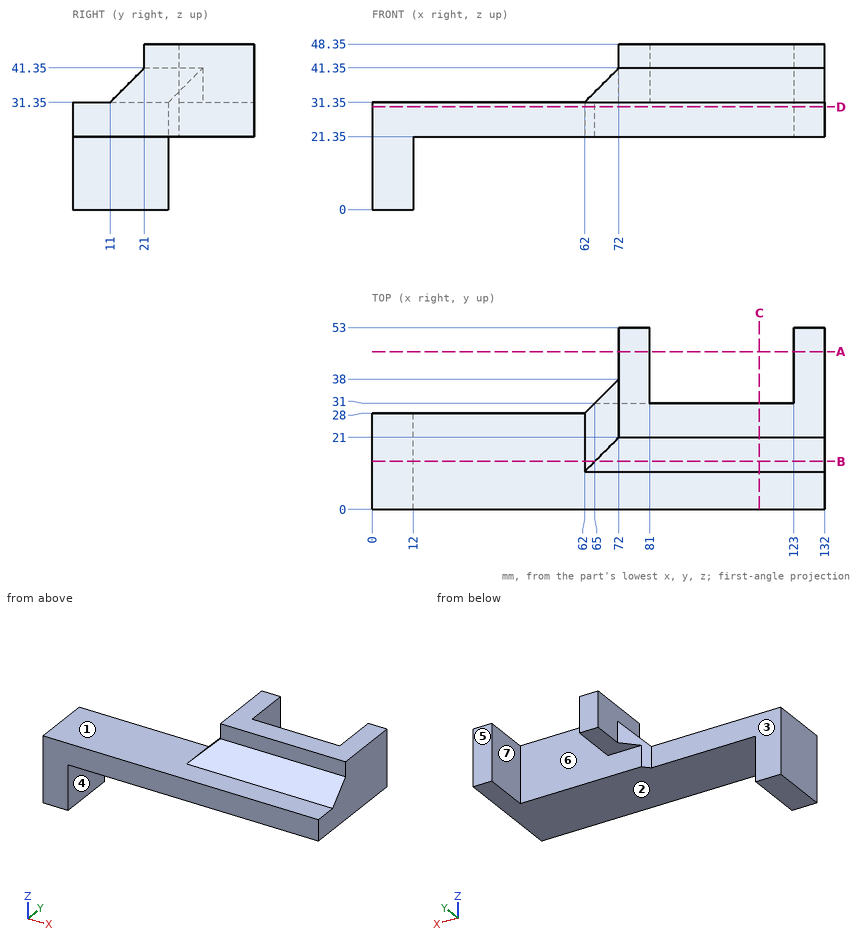
Design review of the part shown in the three views and the two pictorial views. Dimensions are in mm from the part's minimum x, y and z. A direction names the side the tool comes from. Round coordinates to 2 decimals unless told otherwise and drop trailing zeros. Loops run counter-clockwise (first coordinate to the right, second up) from the corner with the lowest first, then second, coordinate; pieces in that order, holes last.
1) Consider section B-B on y = 14. State the section outline as (x, z) points, then the cut area to 3 significant figures.
Values follow:
outline: (0, 0) - (12, 0) - (12, 21.35) - (132, 21.35) - (132, 34.35) - (65, 34.35) - (62, 31.35) - (0, 31.35) - close
area: 1,780 mm2
2) Wall thickness on line 1 along Z through (x, y) = (32, 27.5); line 2 along Z through (x, y) = (9, 6.5); line 3 along X through (y, z) = (23, 43): over which ranges is each line inside the solid? List them lowest first.
Values follow:
line 1: z = 21.35 to 31.35
line 2: z = 0 to 31.35
line 3: x = 72 to 132
3) Consider section C-C on x = 113. State the section outline as (y, z) points.
Values follow:
outline: (0, 21.35) - (31, 21.35) - (31, 48.35) - (21, 48.35) - (21, 41.35) - (11, 31.35) - (0, 31.35) - close
4) Clearance check with flat-ended pins moving along their axes: P1, Ø8.5, axis at x = 88.5, y = 10, coming from the +Z side; P2, Ø7.5, axis at x = 98.5, z = 45.5, coming from the -Y side; P3, Ø13, axis at x = 73, y = 42, coming from the -Z side; P4, Ø2, axis at y = 14, z = 24.5, coming from the -X side. State where each tip first meets the part, or that it passes through.
Values follow:
P1: stops at z = 34.6
P2: stops at y = 21
P3: stops at z = 31.35
P4: stops at x = 0
5) The part is to be moulded in two halves that separate along X. For the marked faces 4, 5, 6 and 7, say which applies: pulls with the +X half, pulls with the -X half, needs draft (parallel to the pull), parting line crosses it, or undercut.
Values follow:
face 4: pulls with the +X half
face 5: needs draft
face 6: undercut
face 7: undercut
6) Consider section A-A on y = 46. State the section outline as (x, z) points, then the cut area to 3 significant figures.
Values follow:
outline: (72, 31.35) - (81, 31.35) - (81, 48.35) - (72, 48.35) - close; (123, 21.35) - (132, 21.35) - (132, 48.35) - (123, 48.35) - close
area: 396 mm2
7) Tool access review of the marked faces 1, 2 and 3: name each direction out of +Z, -Z, +X, -X, +Y, -Y from which nothing blocks a thin tool from reaching the whole face with its end or side.
Values follow:
face 1: +Z, -X, -Y
face 2: -Z, +X, +Y, -Y
face 3: +Z, -Z, -X, +Y
8) Consider section D-D on z = 30. State the section outline as (x, y) points.
Values follow:
outline: (0, 0) - (132, 0) - (132, 53) - (123, 53) - (123, 31) - (65, 31) - (62, 28) - (0, 28) - close
